from build123d import *

# Parameters (mm, degrees)
SKETCH1_W           = 7
SKETCH1_H           = 7
BOSS_EXTRUDE1_DEPTH = 8.4
CHAMFER1_SIZE       = 3.5
CHAMFER1_SIZE2      = 1.27389582
SKETCH2_W           = 2.85
SKETCH2_H           = 4.2
CUT_EXTRUDE1_DEPTH  = 1.8
SKETCH3_R           = 1
CUT_EXTRUDE2_DEPTH  = 4.2
SKETCH4_R           = 1.3
CUT_EXTRUDE3_DEPTH  = 1
SKETCH5_R           = 0.45
BOSS_EXTRUDE2_DEPTH = 4.2
FILLET1_R           = 0.3


with BuildPart() as part:
    # Sketch1 → Boss-Extrude1 (new body)
    with BuildSketch(Plane.XY):
        Rectangle(SKETCH1_W, SKETCH1_H)
    extrude(amount=BOSS_EXTRUDE1_DEPTH)

    # Chamfer1
    chamfer1_edges = [part.edges().sort_by_distance(p)[0] for p in [
        (0, -3.5, 8.4),
    ]]
    chamfer1_side = [part.faces().sort_by_distance(p)[0] for p in [
        (0, -3.5, 4.2),
    ]]
    chamfer(chamfer1_edges, length=CHAMFER1_SIZE, length2=CHAMFER1_SIZE2, reference=chamfer1_side[0])

    # Sketch2 → Cut-Extrude1 (cut)
    with BuildSketch(Plane.XZ.offset(3.5)):
        with Locations((1.725, 2.6)):
            Rectangle(SKETCH2_W, SKETCH2_H)
        with Locations((-1.725, 2.6)):
            Rectangle(SKETCH2_W, SKETCH2_H)
    extrude(amount=-CUT_EXTRUDE1_DEPTH, mode=Mode.SUBTRACT)

    # Sketch3 → Cut-Extrude2 (cut)
    with BuildSketch(Plane.XZ.offset(1.7)):
        with Locations((-1.725, 2.6)):
            Circle(SKETCH3_R)
        with Locations((1.725, 2.6)):
            Circle(SKETCH3_R)
    extrude(amount=-CUT_EXTRUDE2_DEPTH, mode=Mode.SUBTRACT)

    # Sketch4 → Cut-Extrude3 (cut)
    with BuildSketch(Plane.XY.offset(8.4)):
        with Locations((-1.725, 0.5)):
            Circle(SKETCH4_R)
        with Locations((1.725, 0.5)):
            Circle(SKETCH4_R)
    extrude(amount=-CUT_EXTRUDE3_DEPTH, mode=Mode.SUBTRACT)

    # Sketch5 → Boss-Extrude2 (add)
    with BuildSketch(Plane(origin=(0, 0, 0), x_dir=(-1, 0, 0), z_dir=(0, 0, -1))):
        with Locations((-1.75, 0)):
            Circle(SKETCH5_R)
        with Locations((1.75, 0)):
            Circle(SKETCH5_R)
    extrude(amount=BOSS_EXTRUDE2_DEPTH)

    # Fillet1
    fillet1_edges = [part.edges().sort_by_distance(p)[0] for p in [
        (2.2, 0, -4.2),
        (-1.3, 0, -4.2),
    ]]
    fillet(fillet1_edges, radius=FILLET1_R)


solid = part.part
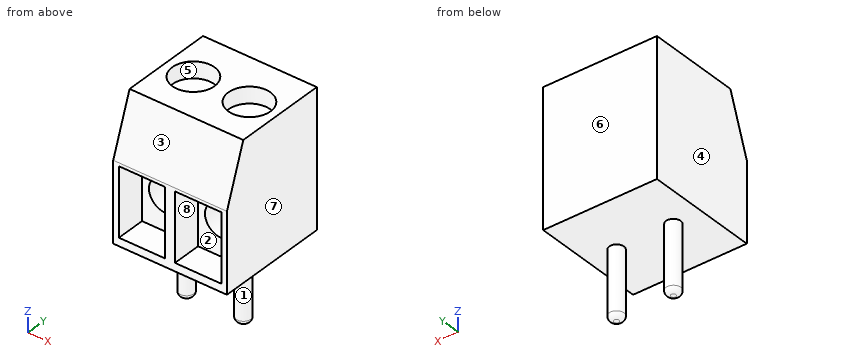
The listing builds one solid part. Answer for the finished solid, in the listing's coordinates (mm). Face numbers are marked on the shaded views. A direction names the side the tool comes from. Round coordinates to 2 decimals unless told otherwise and drop trailing zeros. Order: outer loops, then holes, each group sorted by start corner. A loop starts at its lowest first (then second) coordinate and runs counter-clockwise, first axis right, second up. Notation, with made-up numbers: M 33,-27.5 L 60,-27.5 A23 cw 60,10.5 Z; hole C 19,-0.5 d2. An arc over 180 degrees is marked long. Answer in a Markdown table with one row per item. Add a question column.
1) Flat-ended cylindrical pins translate along their axes: pin 1 Ø0.8 at (x, y) = (1, 0.5) entering from +Z; pin 2 Ø0.5 at (x, y) = (-2, -2.5) entering from -Z; pin 3 Ø1.4 at (x, z) = (2, 3) entering from -Y. Find the tip coordinate at first contact, or state that the pin passes through.
2) The part is cut by section B-B on y = 1. Determine the outline of the cut face in (x, z) (3 decimals), plus the area to 3 significant figures.
3) Which of the six approach directions +Z, -Z, +X, -X, +Y, -Y give full straight-line access (tool end or side, diameter ignored) to the marked faces 1, 2, 3, 4 and 5?
4) The part is cut by section C-C on z = -2.5. Determine the outline of the cut face in (x, y).
5) Consider line 1 along X through (y, z) = (-2.5, 1.25); line 2 along Z through (x, y) = (-2.5, -2); line 3 along Y through (x, z) = (-3, 2). Determine where each line is inside the solid, lowest interval first. Write a range as from..to.
6) The part is cut by section D-D on x = -2.5. Determine the outline of the cut face in (y, z).
7) Determine the mould class of the marked faces 6, 7 and 8 for opening direction X: pulls with the +X half, pulls with the -X half, needs draft (parallel to the pull), parting line crosses it, or undercut.
8) The part is cut by section A-A on z = 2.6. Determine the outline of the cut face in (x, y) (3 decimals).
Findings below:
| question | item | result |
|---|---|---|
| 1 | pin 1 | stops at z = 7.4 |
| 1 | pin 2 | stops at z = 0 |
| 1 | pin 3 | stops at y = -1.7 |
| 2 | outline | M -3.5,0 L 3.5,0 L 3.5,8.4 L 2.925,8.4 L 2.925,7.4 L 0.525,7.4 L 0.525,8.4 L -0.525,8.4 L -0.525,7.4 L -2.925,7.4 L -2.925,8.4 L -3.5,8.4 Z; hole C -1.725,2.6 d2; hole C 1.725,2.6 d2 |
| 2 | area | 47.7 mm² |
| 3 | face 1 | -Z |
| 3 | face 2 | -Y |
| 3 | face 3 | +Z, +X, -X, -Y |
| 3 | face 4 | +Z, -Z, -X, +Y, -Y |
| 3 | face 5 | +Z |
| 4 | outline | C -1.75,0 d0.9; C 1.75,0 d0.9 |
| 5 | line 1 | x = -3.5..-3.15, -0.3..0.3, 3.15..3.5 |
| 5 | line 2 | z = 0..0.5, 4.7..8.4 |
| 5 | line 3 | y = -1.7..3.5 |
| 6 | outline | M -3.5,0 L 3.5,0 L 3.5,8.4 L 1.54,8.4 L 1.54,7.4 L -0.54,7.4 L -0.54,8.4 L -2.23,8.4 L -3.5,4.9 L -3.5,4.7 L -1.7,4.7 L -1.7,3.23 L 2.5,3.23 L 2.5,1.97 L -1.7,1.97 L -1.7,0.5 L -3.5,0.5 Z |
| 7 | face 6 | needs draft |
| 7 | face 7 | pulls with the +X half |
| 7 | face 8 | undercut |
| 8 | outline | M -3.5,-3.5 L -3.15,-3.5 L -3.15,-1.7 L -2.725,-1.7 L -2.725,2.5 L -0.725,2.5 L -0.725,-1.7 L -0.3,-1.7 L -0.3,-3.5 L 0.3,-3.5 L 0.3,-1.7 L 0.725,-1.7 L 0.725,2.5 L 2.725,2.5 L 2.725,-1.7 L 3.15,-1.7 L 3.15,-3.5 L 3.5,-3.5 L 3.5,3.5 L -3.5,3.5 Z |
